```python
from build123d import *

# Parameters (mm, degrees)
SKETCH003_R     = 17.1
PAD001_DEPTH    = 10
SKETCH001_W     = 6
SKETCH001_H     = 4
POCKET_DEPTH    = 50
SKETCH004_R     = 1.9
POCKET001_DEPTH = 20
SKETCH006_R     = 1.9
POCKET002_DEPTH = 20
SKETCH007_R     = 1.45
POCKET003_DEPTH = 20
SKETCH_W        = 7.2
SKETCH_H        = 3.7
POCKET004_DEPTH = 9


with BuildPart() as part:
    # Sketch003 → Pad001 (new body)
    with BuildSketch(Plane.XY):
        Polygon((-40, -40), (-40, 30), (-40, 70), (-6.4034604704, 70), (-6.4034604704, 41.7587995296), (5.3553390593, 30), (35.0538238691, 59.6984848098), (35.0538238691, 70), (69.6984848098, 70), (69.6984848098, 25.0538238692), (40, -4.6446609407), (40, -40), align=None)
        Circle(SKETCH003_R, mode=Mode.SUBTRACT)
    extrude(amount=PAD001_DEPTH)

    # Sketch001 → Pocket (cut)
    with BuildSketch(Plane(origin=(22.3223304704, -22.3223304703, 0), x_dir=(0.7071067812, 0.7071067812, 0), z_dir=(0.7071067812, -0.7071067812, 0))):
        with Locations((30.5, 5)):
            Rectangle(SKETCH001_W, SKETCH001_H)
        with Locations((61.5, 5)):
            Rectangle(SKETCH001_W, SKETCH001_H)
    extrude(amount=-POCKET_DEPTH, mode=Mode.SUBTRACT)

    # Sketch004 → Pocket001 (cut)
    with BuildSketch(Plane(origin=(0, 70, 0), x_dir=(-1, 0, 0), z_dir=(0, 1, 0))):
        with Locations((30, 5)):
            Circle(SKETCH004_R)
        with Locations((-60, 5)):
            Circle(SKETCH004_R)
    extrude(amount=-POCKET001_DEPTH, mode=Mode.SUBTRACT)

    # Sketch006 → Pocket002 (cut)
    with BuildSketch(Plane.XZ.offset(40)):
        with Locations((30, 5)):
            Circle(SKETCH006_R)
        with Locations((-30, 5)):
            Circle(SKETCH006_R)
    extrude(amount=-POCKET002_DEPTH, mode=Mode.SUBTRACT)

    # Sketch007 → Pocket003 (cut)
    with BuildSketch(Plane(origin=(-40, 0, 0), x_dir=(0, -1, 0), z_dir=(-1, 0, 0))):
        with Locations((-15.5, 5)):
            Circle(SKETCH007_R)
        with Locations((15.5, 5)):
            Circle(SKETCH007_R)
    extrude(amount=-POCKET003_DEPTH, mode=Mode.SUBTRACT)

    # Sketch → Pocket004 (cut)
    with BuildSketch(Plane.XY.offset(10)):
        with Locations((-30, -30.15)):
            Rectangle(SKETCH_W, SKETCH_H)
        with Locations((30, -30.15)):
            Rectangle(SKETCH_W, SKETCH_H)
        with Locations((-30, 60.15)):
            Rectangle(SKETCH_W, SKETCH_H)
        with Locations((60, 60.15)):
            Rectangle(SKETCH_W, SKETCH_H)
    extrude(amount=-POCKET004_DEPTH, mode=Mode.SUBTRACT)


solid = part.part
```
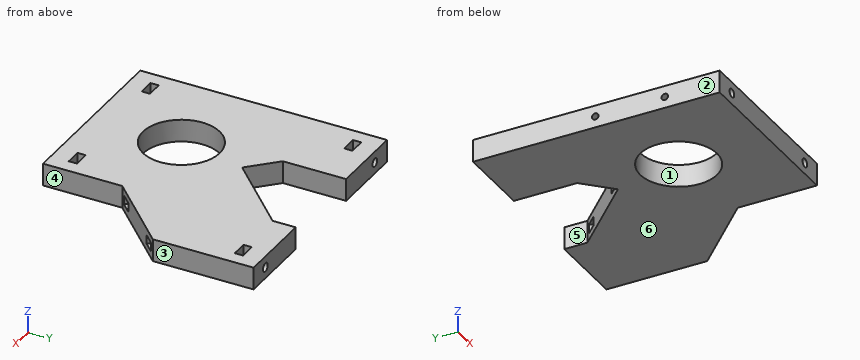
Geometry check sheet. Reference: the model listing, model coordinates, mm. Face numbers are marked on the shaded views. A direction names the side the tool comes from. Coordinates: 2 decimals unless noted, no trailing zeros. Write each loop counter-clockwise with the first axis right and the second up, starting at its lowest first coordinate (ties: lowest second). Pieces come first, ordered by that corner, then holes. Notation, with made-up numbers: M 19,-1 L 61,-1 A31 ccw 61,25 Z; hole C 56,-34 d8. An arc over 180 degrees is marked long. One line per item, written item: value. Start each with the question number.
(1) Depth check by flat-ended pin: pin 1 (1.9 mm diameter, centred on x = 60, y = 60, fed in from +Z); pin 2 (5 mm diameter, centred on y = 21.5, z = 8.5, fed in from +X); pin 3 (6 mm diameter, centred on x = 30, z = 5, fed in from +Y). Enter the tip coordinate at first touch or a pass-through.
(2) Sectioned sample at B-B, the plane y = 51.5. Enter the section's corners in (x, z), and give its area (3 significant figures).
(3) Tool access check on the marked faces 4, 5 and 6. Record the directions out of +Z, -Z, +X, -X, +Y, -Y that give a thin tool (end or side, any length) a straight path to the whole face; none if there is none.
(4) Sectioned sample at A-A, the plane x = -30. State how many separate pieces and enclosed holes the cut face has, and give its area (3 significant figures).
(5) Scan lines: line 1 along Z through (x, y) = (30, -38.5); line 2 along X through (y, z) = (59.5, 8.75); line 3 along X through (y, z) = (28.5, 4.5). Record each from-to range of solid material in increasing order. Write a range as [from, to].
(6) Sectioned sample at D-D, the plane x = 0. Enter the section's corners in (y, z), and give its area (3 significant figures).
(7) Sectioned sample at C-C, the plane y = 5.5. Enter the section's corners in (x, z), and give its area (3 significant figures).
(8) Release check for a two-part mould opening along X. For the marked faces 1, 2 and 3 record: released by +X, released by -X, zero draft, split by the parting line, or undercut.
Filled sheet:
1. pin 1: z = 1
1. pin 2: x = 68.64
1. pin 3: y = 56.88
2. outline: M -40,0 L -6.4,0 L -6.4,10 L -40,10 Z; M 26.86,0 L 69.7,0 L 69.7,10 L 26.86,10 Z; hole C -30,5 d3.8; hole M 31.23,3 L 39.72,3 L 39.72,7 L 31.23,7 Z; hole C 60,5 d3.8
2. area: 708 mm²
3. face 4: +Z, -Z, +X, -Y
3. face 5: +Z, -Z, +Y
3. face 6: -Z, +X, -X, +Y, -Y
4. separate pieces: 3
4. enclosed holes: 2
4. area: 896 mm²
5. line 1: [0, 3.1], [6.9, 10]
5. line 2: [-40, -33.6], [-26.4, -6.4], [34.86, 56.4], [63.6, 69.7]
5. line 3: [-40, 10.39], [18.88, 54.23], [62.72, 69.7]
6. outline: M -40,0 L -17.1,0 L -17.1,10 L -40,10 Z; M 17.1,0 L 35.36,0 L 35.36,10 L 17.1,10 Z
6. area: 412 mm²
7. outline: M -40,0 L -16.19,0 L -16.19,10 L -40,10 Z; M 16.19,0 L 50.14,0 L 50.14,10 L 16.19,10 Z; hole M 33.39,3 L 41.88,3 L 41.88,7 L 33.39,7 Z
7. area: 544 mm²
8. face 1: undercut
8. face 2: released by -X
8. face 3: released by +X
